Could you check a few things on this model? Use its own coordinates, in mm. Face numbers are marked on the shaded views. A direction names the side the tool comes from. Coordinates: 2 decimals unless noted, no trailing zeros. Write each loop counter-clockwise with the first axis right and the second up, starting at its lowest first coordinate (ties: lowest second). Pieces come first, ordered by that corner, then holes. Notation, with made-up numbers: (41, 85.25) - (67, 85.25) arc R22 cw to (67, 111.25) - close; hole circle Ø4 at (22.25, 20). An arc over 180 degrees is marked (long way). Answer as a JSON object with one key per item and string values. Group by question number.
1) Please list where these lines run through material, in increasing order: line 1 along Z through (x, y) = (-0.9, 7.5); line 2 along X through (y, z) = (-4.5, -6.25); line 3 along Z through (x, y) = (0.95, 3.25).
2) Will these pins go through, and if not, where does the flat tip stop? pin 1 Ø7.5 at (y, z) = (-4, 0) entering from -X; pin 2 Ø1 at (x, y) = (0.5, -3) entering from +Z.
3) We'd pull the mould along Z, two halves only. Please class the marked faces 3, 4 and 5: released by +Z, released by -Z, zero draft, split by the parting line, or undercut.
4) If we section it at B-B (z = 0): Write out the boundary of the cut face in (x, y).
5) If we section it at C-C (x = -2.1): Write out the boundary of the cut face in (y, z).
6) If we section it at D-D (x = 1.3): Write out the boundary of the cut face in (y, z), plus the area to 3 significant figures.
7) If we section it at A-A (y = 0): Write out the boundary of the cut face in (x, z), plus the area to 3 significant figures.
8) On a 3-axis mill with a long thin cutter (end or side, diameter ignored), from which of +Z, -Z, +X, -X, +Y, -Y can I reach the whole of each face in a straight line? I mean the marked faces 1 and 2. Say none if no direction works.
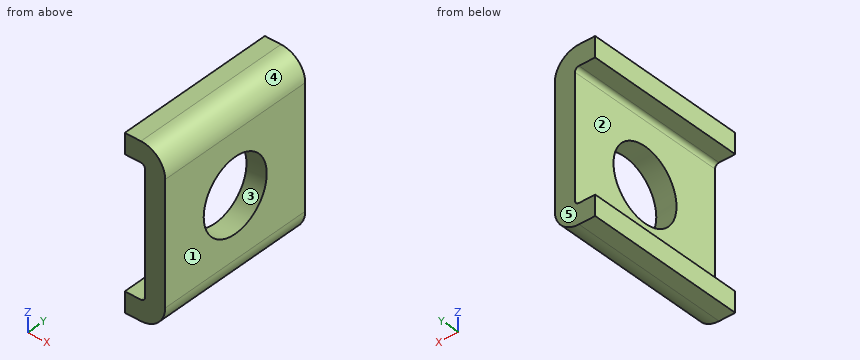
```python
from build123d import *

# Parameters (mm, degrees)
F1_DEPTH      = 10
F1_DEPTH_BACK = 10
F4_D          = 9


with BuildPart() as f1:
    # F0 (on Front) → F1 (new body, two sides)
    with BuildSketch(Plane.XZ) as f1_sk:
        with BuildLine():
            Line((0, 0), (2.5, 0))
            Line((2.5, 0), (2.5, 7.5))
            ThreePointArc((2.5, 7.5), (1.62132, 9.62132), (-0.5, 10.5))
            Line((-0.5, 10.5), (-2.5, 10.5))
            Line((-2.5, 10.5), (-2.5, 8))
            Line((-2.5, 8), (-0.5, 8))
            ThreePointArc((-0.5, 8), (-0.146447, 7.853553), (0, 7.5))
            Line((0, 7.5), (0, 0))
        make_face()
    extrude(amount=F1_DEPTH)
    extrude(f1_sk.sketch, amount=-F1_DEPTH_BACK)

    # F2: F1 across face


with BuildPart() as f1_1:
    add(f1.part)
    add(f1.part.mirror(Plane(origin=(1.25, 0, 0), x_dir=(1, 0, 0), z_dir=(0, 0, -1))))

    # F4 (through all)
    with Locations(Plane.YZ.offset(2.5)):
        with Locations((0, 0)):
            Hole(F4_D / 2)


solid = f1_1.part
```
Here are the results:
{
 "1": {"line 1": "z = -10.5 to -8, 8 to 10.5", "line 2": "x = 0 to 2.5", "line 3": "z = -10.13 to -3.11, 3.11 to 10.13"},
 "2": {"pin 1": "stops at x = 0", "pin 2": "stops at z = 10.46"},
 "3": {"face 3": "undercut", "face 4": "released by +Z", "face 5": "zero draft"},
 "4": {"outline": "(0, -10) - (2.5, -10) - (2.5, -4.5) - (0, -4.5) - close; (0, 4.5) - (2.5, 4.5) - (2.5, 10) - (0, 10) - close"},
 "5": {"outline": "(-10, -10.5) - (10, -10.5) - (10, -8) - (-10, -8) - close; (-10, 8) - (10, 8) - (10, 10.5) - (-10, 10.5) - close"},
 "6": {"outline": "(-10, -9.9) - (10, -9.9) - (10, 9.9) - (-10, 9.9) - close; hole circle Ø9 at (0, 0)", "area": "332 mm²"},
 "7": {"outline": "(-2.5, -10.5) - (-0.5, -10.5) arc R3 ccw to (2.5, -7.5) - (2.5, -4.5) - (0, -4.5) - (0, -7.5) arc R0.5 cw to (-0.5, -8) - (-2.5, -8) - close; (-2.5, 8) - (-0.5, 8) arc R0.5 cw to (0, 7.5) - (0, 4.5) - (2.5, 4.5) - (2.5, 7.5) arc R3 ccw to (-0.5, 10.5) - (-2.5, 10.5) - close", "area": "38.7 mm²"},
 "8": {"face 1": "+Z, -Z, +X, +Y, -Y", "face 2": "-X, +Y, -Y"}
}
